```python
from build123d import *

# Parameters (mm, degrees)
BOSS_EXTRUDE1_DEPTH    = 3
SKETCH2_W              = 0.9
SKETCH2_H              = 15.45
BOSS_EXTRUDE2_DEPTH    = 3
SPLIT1_DEPTH           = 3
SPLIT1_START           = -36.35
SPLIT1_2_OUTLINE_W     = 16.25
SPLIT1_2_OUTLINE_H     = 3
SPLIT1_2_DEPTH         = 0.9
SPLIT1_START_2         = -35.45
SPLIT1_3_OUTLINE_W     = 0.8
SPLIT1_3_OUTLINE_H     = 3
SPLIT1_3_DEPTH         = 7.95
SPLIT1_4_DEPTH         = 3
BODY_MOVE_COPY13_ANGLE = 180
BODY_MOVE_COPY17_ANGLE = 180


# Read off the part's stored shape, not the designer's step: Split1
with BuildPart() as part:
    # Sketch1 → Boss-Extrude1 (new body)
    with BuildSketch(Plane(origin=(0, 0, 0), x_dir=(0, 1, 0), z_dir=(0, 0, 1))):
        with BuildLine():
            Line((0, 0), (-16.25, 0))
            add(Edge.make_bspline(
                [(-16.25, 0), (-9.683887405, 4.589558491), (-5.164437434, 10.570069252), (-2.691650088, 17.941532282)],
                knots=[0, 0, 0, 0, 0.866320649, 0.866320649, 0.866320649, 0.866320649], degree=3))
            Line((-2.691650088, 17.941532282), (-16.25, 8.447873633))
            Line((-16.25, 8.447873633), (-16.25, 18.197873462))
            Line((-16.25, 18.197873462), (-1.693141934, 26.602279385))
            Line((-1.693141934, 26.602279385), (-16.25, 26.602279385))
            Line((-16.25, 26.602279385), (-16.25, 45.197720615))
            Line((-16.25, 45.197720615), (-1.693141934, 45.197720615))
            Line((-1.693141934, 45.197720615), (-16.25, 53.602126538))
            Line((-16.25, 53.602126538), (-16.25, 63.352126367))
            Line((-16.25, 63.352126367), (-2.691650088, 53.858467718))
            add(Edge.make_bspline(
                [(-16.25, 71.8), (-9.683887405, 67.210441509), (-5.164437434, 61.229930748), (-2.691650088, 53.858467718)],
                knots=[0, 0, 0, 0, 0.866320649, 0.866320649, 0.866320649, 0.866320649], degree=3))
            Line((-16.25, 71.8), (0, 71.8))
            Line((0, 71.8), (0, 70.499844847))
            Line((0, 70.499844847), (-13.214812034, 70.499844847))
            add(Edge.make_bspline(
                [(-13.214812034, 70.499844847), (-7.643374044, 65.864497023), (-3.799959359, 60.162821742), (-1.68456798, 53.394819004)],
                knots=[0, 0, 0, 0, 0.803721546, 0.803721546, 0.803721546, 0.803721546], degree=3))
            Line((-1.68456798, 53.394819004), (0, 53.394819004))
            Line((0, 53.394819004), (0, 51.800000008))
            Line((0, 51.800000008), (-1.146610933, 51.800000008))
            Line((-1.146610933, 51.800000008), (-15.450000067, 61.815340728))
            Line((-15.450000067, 61.815340728), (-15.450000067, 54.064006792))
            Line((-15.450000067, 54.064006792), (-1.293141934, 45.890540938))
            Line((-1.293141934, 45.890540938), (0, 45.9))
            Line((0, 45.9), (0, 44.3))
            Line((0, 44.3), (-15.45, 44.3))
            Line((-15.45, 44.3), (-15.45, 27.5))
            Line((-15.45, 27.5), (0, 27.5))
            Line((0, 27.5), (0, 25.9))
            Line((0, 25.9), (-1.293141934, 25.909459062))
            Line((-1.293141934, 25.909459062), (-15.450000067, 17.735993208))
            Line((-15.450000067, 17.735993208), (-15.450000067, 9.984659272))
            Line((-15.450000067, 9.984659272), (-1.146610933, 19.999999992))
            Line((-1.146610933, 19.999999992), (0, 19.999999992))
            Line((0, 19.999999992), (0, 18.405180996))
            Line((0, 18.405180996), (-1.68456798, 18.405180996))
            add(Edge.make_bspline(
                [(-13.214812034, 1.300155153), (-7.643374044, 5.935502977), (-3.799959359, 11.637178258), (-1.68456798, 18.405180996)],
                knots=[0, 0, 0, 0, 0.803721546, 0.803721546, 0.803721546, 0.803721546], degree=3))
            Line((-13.214812034, 1.300155153), (0, 1.300155153))
            Line((0, 1.300155153), (0, 0))
        make_face()
    extrude(amount=BOSS_EXTRUDE1_DEPTH)

    # Sketch2 → Boss-Extrude2 (add)
    with BuildSketch(Plane.XY.offset(3)):
        with Locations((-35.9, -7.725)):
            Rectangle(SKETCH2_W, SKETCH2_H)
    extrude(amount=-BOSS_EXTRUDE2_DEPTH)

    # Split1 outline → Split1 (cut)
    with BuildSketch(Plane.XY):
        with BuildLine():
            Line((-53.394819004, 0), (-53.394819004, -1.68456798))
            add(Edge.make_bspline(
                [(-53.394819004, -1.68456798), (-60.162821742, -3.799959359), (-65.864497023, -7.643374044), (-70.499844847, -13.214812034)],
                knots=[0, 0, 0, 0, 0.803721546, 0.803721546, 0.803721546, 0.803721546], degree=3))
            Line((-70.499844847, -13.214812034), (-70.499844847, 0))
            Line((-70.499844847, 0), (-71.8, 0))
            Line((-71.8, 0), (-71.8, -16.25))
            add(Edge.make_bspline(
                [(-71.8, -16.25), (-67.210441509, -9.683887405), (-61.229930748, -5.164437434), (-53.858467718, -2.691650088)],
                knots=[0, 0, 0, 0, 0.866320649, 0.866320649, 0.866320649, 0.866320649], degree=3))
            Line((-53.858467718, -2.691650088), (-63.352126367, -16.25))
            Line((-63.352126367, -16.25), (-53.602126538, -16.25))
            Line((-53.602126538, -16.25), (-45.197720615, -1.693141934))
            Line((-45.197720615, -1.693141934), (-45.197720615, -16.25))
            Line((-45.197720615, -16.25), (-27.5, -16.25))
            Line((-27.5, -16.25), (-27.5, -15.45))
            Line((-27.5, -15.45), (-35.45, -15.45))
            Line((-35.45, -15.45), (-35.45, 0))
            Line((-35.45, 0), (-36.35, 0))
            Line((-36.35, 0), (-36.35, -15.45))
            Line((-36.35, -15.45), (-44.3, -15.45))
            Line((-44.3, -15.45), (-44.3, 0))
            Line((-44.3, 0), (-45.9, 0))
            Line((-45.9, 0), (-45.890540938, -1.293141934))
            Line((-45.890540938, -1.293141934), (-54.064006792, -15.450000067))
            Line((-54.064006792, -15.450000067), (-61.815340728, -15.450000067))
            Line((-61.815340728, -15.450000067), (-51.800000008, -1.146610933))
            Line((-51.800000008, -1.146610933), (-51.800000008, 0))
            Line((-51.800000008, 0), (-53.394819004, 0))
        make_face()
    extrude(amount=SPLIT1_DEPTH, mode=Mode.SUBTRACT)


with BuildPart() as body_2:
    # Split1 2 outline → Split1 2 (new body)
    with BuildSketch(Plane.YZ.offset(SPLIT1_START)):
        with Locations((-8.125, 1.5)):
            Rectangle(SPLIT1_2_OUTLINE_W, SPLIT1_2_OUTLINE_H)
    extrude(amount=SPLIT1_2_DEPTH)

    # Split1 3 outline → Split1 3 (add)
    with BuildSketch(Plane.YZ.offset(SPLIT1_START_2)):
        with Locations((-15.85, 1.5)):
            Rectangle(SPLIT1_3_OUTLINE_W, SPLIT1_3_OUTLINE_H)
    extrude(amount=SPLIT1_3_DEPTH)


with BuildPart() as body_3:
    # Split1 4 outline → Split1 4 (new body)
    with BuildSketch(Plane.XY):
        with BuildLine():
            Line((-36.35, -16.25), (-36.35, -15.45))
            Line((-36.35, -15.45), (-44.3, -15.45))
            Line((-44.3, -15.45), (-44.3, 0))
            Line((-44.3, 0), (-45.9, 0))
            Line((-45.9, 0), (-45.890540938, -1.293141934))
            Line((-45.890540938, -1.293141934), (-54.064006792, -15.450000067))
            Line((-54.064006792, -15.450000067), (-61.815340728, -15.450000067))
            Line((-61.815340728, -15.450000067), (-51.800000008, -1.146610933))
            Line((-51.800000008, -1.146610933), (-51.800000008, 0))
            Line((-51.800000008, 0), (-53.394819004, 0))
            Line((-53.394819004, 0), (-53.394819004, -1.68456798))
            add(Edge.make_bspline(
                [(-53.394819004, -1.68456798), (-60.162821742, -3.799959359), (-65.864497023, -7.643374044), (-70.499844847, -13.214812034)],
                knots=[0, 0, 0, 0, 0.803721546, 0.803721546, 0.803721546, 0.803721546], degree=3))
            Line((-70.499844847, -13.214812034), (-70.499844847, 0))
            Line((-70.499844847, 0), (-71.8, 0))
            Line((-71.8, 0), (-71.8, -16.25))
            add(Edge.make_bspline(
                [(-71.8, -16.25), (-67.210441509, -9.683887405), (-61.229930748, -5.164437434), (-53.858467718, -2.691650088)],
                knots=[0, 0, 0, 0, 0.866320649, 0.866320649, 0.866320649, 0.866320649], degree=3))
            Line((-53.858467718, -2.691650088), (-63.352126367, -16.25))
            Line((-63.352126367, -16.25), (-53.602126538, -16.25))
            Line((-53.602126538, -16.25), (-45.197720615, -1.693141934))
            Line((-45.197720615, -1.693141934), (-45.197720615, -16.25))
            Line((-45.197720615, -16.25), (-36.35, -16.25))
        make_face()
    extrude(amount=SPLIT1_4_DEPTH)


with BuildPart() as body_3_1:
    # Body-Move/Copy11: moved
    add(body_3.part.moved(Location((-8.85, 0, 0))))


with BuildPart() as body_2_1:
    # Body-Move/Copy12: moved
    add(body_2.part.moved(Location((-8.85, 0, 0))))


with BuildPart() as body_2_2:
    # Body-Move/Copy13: moved
    add(body_2_1.part.rotate(Axis((0, -8.125, 1.5), (1, 0, 0)), BODY_MOVE_COPY13_ANGLE))


with BuildPart() as body_4:
    # Body-Move/Copy14: copy of body 2
    add(body_2_2.part.moved(Location((8.85, 0, 0))))


with BuildPart() as body_4_1:
    # Body-Move/Copy17: moved
    add(body_4.part.rotate(Axis((0, -8.125, 1.5), (1, 0, 0)), BODY_MOVE_COPY17_ANGLE))


with BuildPart() as body_3_2:
    add(body_3_1.part)

    # Combine1: union body 4, body 2, part
    add(body_4_1.part)
    add(body_2_2.part)
    add(part.part)


solid = body_3_2.part
```
The listing builds one solid part. Answer for the finished solid, in the listing's coordinates (mm). A direction names the side the tool comes from. Coordinates: 2 decimals unless noted, no trailing zeros. Loops run counter-clockwise (first coordinate to the right, second up) from the corner with the lowest first, then second, coordinate; pieces in that order, holes last. Notation, with made-up numbers: (16.5, -23) - (64.5, -23) arc R23 ccw to (64.5, 11) - close; hole circle Ø2 at (81.5, 21.25). An arc over 180 degrees is marked (long way). Use a Markdown table: item, result. Add a question column.
1) The part is cut by section C-C, the plane x = -47. Give the vertices of the cut face in (y, z).
2) For faces 4 (the flat face through (-53.15, -8, 1)), 5 (the flat face through (-26.602, -9, 1)), 6 (the flat face through (-13.26, -9.38, 1.48)), determine the directions among +Z, -Z, +X, -X, +Y, -Y from which every point of the face is accessible in a straight line to the end or side of a thin tool.
3) The part is cut by section A-A, the plane x = -66. State how many separate pieces and enclosed holes the cut face has, and give its area (3 significant figures).
4) The mould has two halves that part along Y. Classify faces 1 (the flat face through (-35.45, -8, 2)), 2 (the flat face through (-49, -16.25, 2)), 3 (the flat face through (-14.92, -8.4, 1.48)): released by +Y, released by -Y, zero draft, split by the parting line, or undercut.
5) Find the intervals of material crossed by line 1 (Y direction, x = -65.5, z = 1); line 2 (Y direction, x = -70.5, z = 2.3); line 3 (Y direction, x = -40.5, z = 2.7), in increasing order.
6) Given pin 1 (0.9 mm diameter, centred on x = -67, z = 1.5, fed in from +Y), flat-ended and moving along its own axis, determine where the tip first touches the part or whether it passes through.
Here are the results:
| question | item | result |
|---|---|---|
| 1 | outline | (-16.25, 0) - (-15.45, 0) - (-15.45, 3) - (-16.25, 3) - close |
| 2 | face 4 | +Z, -Z, +Y |
| 2 | face 5 | +Z, -Z, -Y |
| 2 | face 6 | +Z, -Z |
| 3 | separate pieces | 3 |
| 3 | enclosed holes | 0 |
| 3 | area | 9.25 mm^2 |
| 4 | face 1 | zero draft |
| 4 | face 2 | released by -Y |
| 4 | face 3 | undercut |
| 5 | line 1 | y = -16.25 to -15.45, -8.07 to -6.68, -3.75 to -2.87 |
| 5 | line 2 | y = -16.25 to -15.45, -15.21 to -13.82, -6.39 to -5.44 |
| 5 | line 3 | y = -0.8 to 0 |
| 6 | pin 1 | stops at y = -3.33 |
